Read the model definition and answer for the solid it produces. Units are mm, in the model's axes. Face numbers are marked on the shaded views. A direction names the side the tool comes from. Coordinates: 2 decimals unless noted, no trailing zeros. Order: outer loops, then holes, each group sorted by start corner. A loop starts at its lowest first (then second) coordinate and runs counter-clockwise, first axis right, second up. Notation, with made-up numbers: M 20.5,-4.75 L 35.5,-4.75 A9 ccw 35.5,0.25 Z; hole C 83.25,-29 d3. An arc over 180 degrees is marked long. One line per question, with ' | ' between items. Start each with the question number.
1) Find section B-B, the plane x = 6.5. Write down the section's boundary in (y, z).
2) A tool of negligible diameter and unlimited length cuts with its end or side. For the marked faces 1, 2 and 3, from which of +Z, -Z, +X, -X, +Y, -Y can it reach the whole face along a straight path? Write none if from no direction.
3) Find section C-C, the plane z = 3.5. Write down the section's boundary in (x, y), plus the area to 3 significant figures.
4) Consider probe 1 along Z at (x, y) = (-6.5, -1.1); probe 2 along X at (y, z) = (-1, -4); probe 3 along Z at (x, y) = (6, -0.95). Determine where each line is inside the solid, lowest interval first.
5) Given P1, Ø1, axis at x = -10, y = -0.5, coming from the +Z side; P2, Ø0.6, axis at x = -10, y = -1, coming from the -Z side, each flat-ended and moving along its own axis, determine where each tip first touches the part or whether it passes through.
6) The mould has two halves that part along Z. Classify the marked faces 4, 5 and 6: +Z half, -Z half, draft (parallel to the pull), parting line (faces both ways), or undercut.
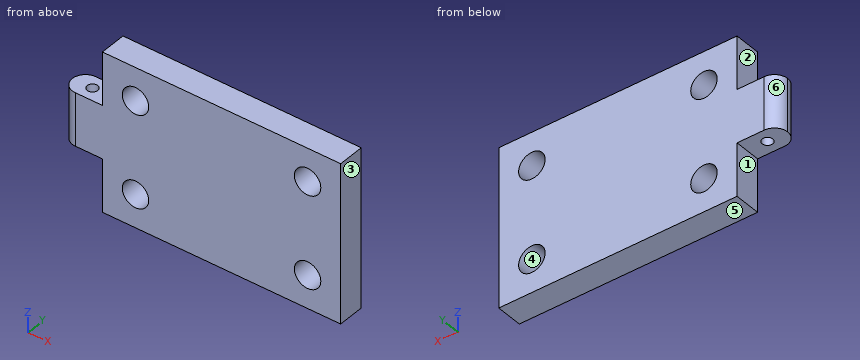
from build123d import *

# Parameters (mm, degrees)
F0_W     = 3.05
F0_H     = 4
F1_DEPTH = 2
F2_R     = 0.4
F3_DEPTH = 25
F4_R     = 1
F5_DEPTH = 25
F6_R     = 0.99999


# Not quite as in the source:
# - a fillet or chamfer is up to 0.001 mm smaller than in the source, because OpenCascade refuses the exact size


with BuildPart() as f1:
    # F0 (on Front) → F1 (new body)
    with BuildSketch(Plane.XZ):
        Polygon((9, -6), (9, 6), (-9, 6), (-9, 2), (-5.95, 2), (-5.95, -2), (-9, -2), (-9, -6), align=None)
        with Locations((-7.475, 0)):
            Rectangle(F0_W, F0_H)
        with Locations((-10.525, 0)):
            Rectangle(F0_W, F0_H)
    extrude(amount=F1_DEPTH)

    # F2 (on face) → F3 (cut)
    with BuildSketch(Plane(origin=(0, 0, -2), x_dir=(1, 0, 0), z_dir=(0, 0, -1))):
        with Locations((-10.525, 1)):
            Circle(F2_R)
    extrude(amount=-F3_DEPTH, mode=Mode.SUBTRACT)

    # F4 (on face) → F5 (cut)
    with BuildSketch(Plane.XZ.offset(2)):
        with Locations((-6.5, 3.5)):
            Circle(F4_R)
        with Locations((6.5, 3.5)):
            Circle(F4_R)
        with Locations((6.5, -3.5)):
            Circle(F4_R)
        with Locations((-6.5, -3.5)):
            Circle(F4_R)
    extrude(amount=-F5_DEPTH, mode=Mode.SUBTRACT)

    # F6 (radius 1 in the source; OpenCascade refuses exactly that, so slightly less here)
    f6_edges = [f1.edges().sort_by_distance(p)[0] for p in [
        (-12.05, -2, 0),
        (-12.05, 0, 0),
    ]]
    fillet(f6_edges, radius=F6_R)


solid = f1.part
Report:
1) outline: M -2,-6 L 0,-6 L 0,-4.5 L -2,-4.5 Z; M -2,-2.5 L 0,-2.5 L 0,2.5 L -2,2.5 Z; M -2,4.5 L 0,4.5 L 0,6 L -2,6 Z
2) face 1: -Z, -X, +Y, -Y | face 2: +Z, -X, +Y, -Y | face 3: +Z, -Z, +X, +Y, -Y
3) outline: M -9,-2 L -7.5,-2 L -7.5,0 L -9,0 Z; M -5.5,-2 L 5.5,-2 L 5.5,0 L -5.5,0 Z; M 7.5,-2 L 9,-2 L 9,0 L 7.5,0 Z | area: 28.0 mm^2
4) probe 1: z = -6 to -4.5, -2.5 to 2.5, 4.5 to 6 | probe 2: x = -9 to -7.37, -5.63 to 5.63, 7.37 to 9 | probe 3: z = -6 to -4.37, -2.63 to 2.63, 4.37 to 6
5) P1: stops at z = 2 | P2: stops at z = -2
6) face 4: undercut | face 5: -Z half | face 6: draft
